from build123d import *

# Parameters (mm, degrees)
REVOLVE1_ANGLE     = 180
SKETCH2_R          = 10.45
CUT_EXTRUDE1_DEPTH = 166.061473397


with BuildPart() as part:
    # Sketch1 → Revolve1 (revolve)
    with BuildSketch(Plane.XY):
        Polygon((-45, 0), (-45, 152.3), (-42, 152.3), (-42, 137.3), (-41, 137.3), (-41, 15), (-43, 15), (-43, 0), align=None)
    revolve(axis=Axis((0, 0, 0), (0, 1, 0)), revolution_arc=REVOLVE1_ANGLE)

    # Sketch2 → Cut-Extrude1 (cut, through all)
    with BuildSketch(Plane(origin=(0, 0, 0), x_dir=(0, 0, -1), z_dir=(1, 0, 0))):
        with Locations((0, 40.3)):
            Circle(SKETCH2_R)
        with Locations((0, 91.5)):
            Circle(SKETCH2_R)
    extrude(amount=-CUT_EXTRUDE1_DEPTH, mode=Mode.SUBTRACT)


solid = part.part
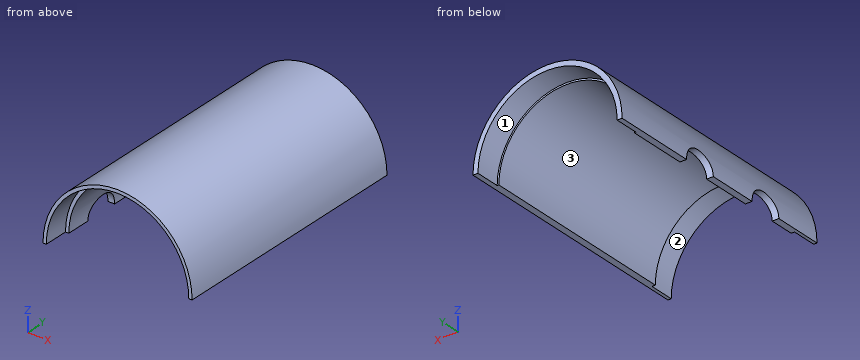
CAD build for the part. Positions are in the model's coordinates, mm. Face numbers are marked on the shaded views. A direction names the side the tool comes from. Give positions to 0.01 mm unless a question says otherwise; leave off trailing zeros. Loops run counter-clockwise (first coordinate to the right, second up) from the corner with the lowest first, then second, coordinate; pieces in that order, holes last. Notation, with made-up numbers: M 28,43 L 72,43 A20 ccw 72,65 Z; hole C 28.25,32 d1. An arc over 180 degrees is marked long. One line per question, with ' | ' between items. Start each with the question number.
1. Flat gauge pins, fed straight in: pin 1 (4 mm diameter, centred on x = 2.5, y = 68.5, fed in from +Z); pin 2 (6 mm diameter, centred on x = 6, y = 77.5, fed in from +Z); pin 3 (5 mm diameter, centred on x = -8.5, y = 73, fed in from +Z). Where does each tip first touch, or does it go through?
2. Saw through at B-B on z = 6. Give the cut face in (x, y), plus the area to 3 significant figures.
3. Saw through at C-C on x = 0. Give the cut face in (y, z), plus the area to 3 significant figures.
4. 3-axis set-ups, long thin cutter, end or side, ignore diameter. For the marked faces 1, 2 and 3: which of +Z, -Z, +X, -X, +Y, -Y reach the whole face in a straight line?
5. Probe L1, parallel to X at y = 121.5, z = 11; L2, parallel to X at y = 46, z = 15.5; L3, parallel to Z at x = -20.5, y = 78. List the from-to ranges inside material, lowest first. Write a range as from..to.
6. Saw through at A-A on z = 18.5. Give the cut face in (x, y).
7. Saw through at D-D on y = 59.5. Give the cut face in (x, z), plus the area to 3 significant figures.
Result sheet:
1) pin 1: stops at z = 45 | pin 2: stops at z = 44.9 | pin 3: stops at z = 44.6
2) outline: M -44.6,0 L -42.58,0 L -42.58,15 L -40.56,15 L -40.56,31.74 L -44.6,31.74 Z; M -44.6,48.86 L -40.56,48.86 L -40.56,82.94 L -44.6,82.94 Z; M -44.6,100.06 L -40.56,100.06 L -40.56,137.3 L -41.57,137.3 L -41.57,152.3 L -44.6,152.3 Z; M 40.56,15 L 42.58,15 L 42.58,0 L 44.6,0 L 44.6,152.3 L 41.57,152.3 L 41.57,137.3 L 40.56,137.3 Z | area: 1,000 mm^2
3) outline: M 0,43 L 15,43 L 15,41 L 137.3,41 L 137.3,42 L 152.3,42 L 152.3,45 L 0,45 Z | area: 564 mm^2
4) face 1: -Z, +Y | face 2: -Z, -Y | face 3: -Z, +Y, -Y
5) L1: x = -43.63..-39.5, 39.5..43.63 | L2: x = -42.25..-37.96, 37.96..42.25 | L3: z = 35.51..40.06
6) outline: M -41.02,0 L -38.82,0 L -38.82,15 L -36.59,15 L -36.59,137.3 L -37.71,137.3 L -37.71,152.3 L -41.02,152.3 Z; M 36.59,15 L 38.82,15 L 38.82,0 L 41.02,0 L 41.02,152.3 L 37.71,152.3 L 37.71,137.3 L 36.59,137.3 Z
7) outline: M -45,0 L -41,0 A41 cw 41,0 L 45,0 A45 ccw Z | area: 540 mm^2
